Answer from the drawing. Dimensions are ordinates in mm from the lowest x, y and z of the part. Round coordinates to 2 decimals unless told otherwise and drop trailing zeros. Write each loop counter-clockwise with the first axis right and the second up, starting at its lowest first coordinate (ties: lowest second). Pieces come first, ordered by that corner, then holes. Notation, with made-up numbers: (1.5, 30) - (18.5, 30) arc R25 ccw to (18.5, 52) - close; hole circle Ø5 at (56.5, 75.5). An arc over 180 degrees is marked (long way). Answer in a Markdown table with one row per item.
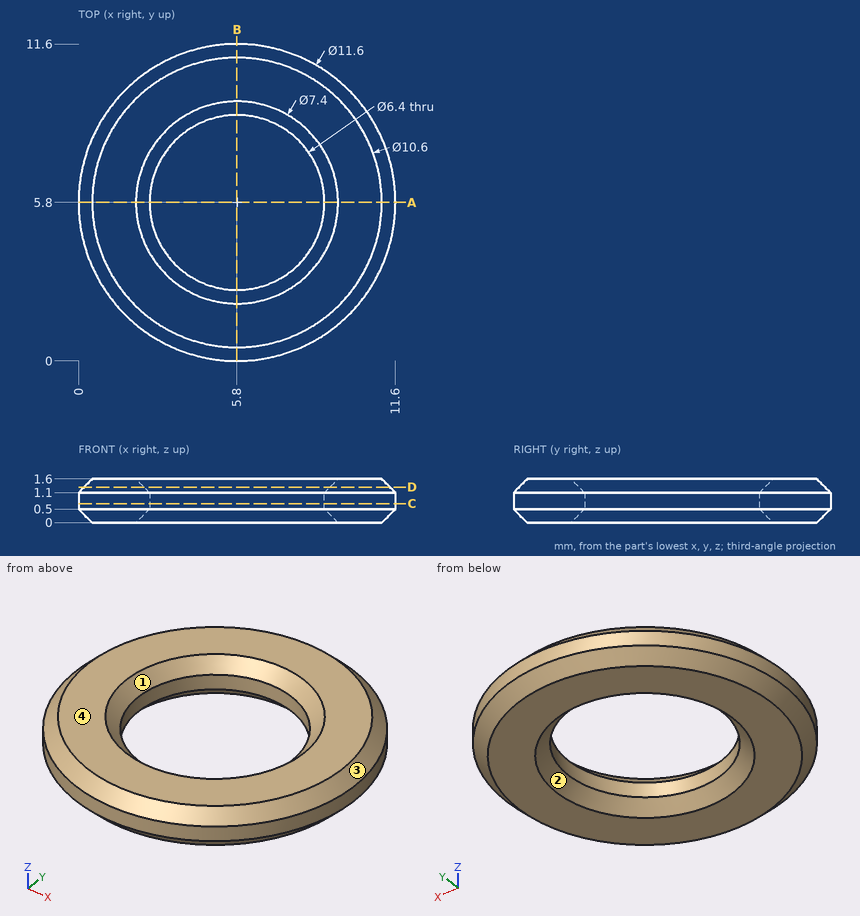
(1) For a pull along X with two mould halves and no side action, classify the marked faces 1, 2, 3 and 4 as pulls with the +X half, pulls with the -X half, needs draft (parallel to the pull), parting line crosses it, or undercut.
Checked values:
| item | result |
|---|---|
| face 1 | undercut |
| face 2 | undercut |
| face 3 | parting line crosses it |
| face 4 | needs draft |
(2) Section C-C (z = 0.7) is taken. Give the vertices of the cut face in (x, y).
Checked values:
| item | result |
|---|---|
| outline | circle Ø11.6 at (5.8, 5.8); hole circle Ø6.4 at (5.8, 5.8) |
(3) Section D-D (z = 1.3) is taken. Give the vertices of the cut face in (x, y), and give its area (3 significant figures).
Checked values:
| item | result |
|---|---|
| outline | circle Ø11.2 at (5.8, 5.8); hole circle Ø6.8 at (5.8, 5.8) |
| area | 62.2 mm2 |
(4) Section A-A (y = 5.8) is taken. Give the vertices of the cut face in (x, z).
Checked values:
| item | result |
|---|---|
| outline | (0, 0.5) - (0.5, 0) - (2.1, 0) - (2.6, 0.5) - (2.6, 1.1) - (2.1, 1.6) - (0.5, 1.6) - (0, 1.1) - close; (9, 0.5) - (9.5, 0) - (11.1, 0) - (11.6, 0.5) - (11.6, 1.1) - (11.1, 1.6) - (9.5, 1.6) - (9, 1.1) - close |
(5) Find the intervals of material crossed by line 1 (Y direction, x = 5.8, z = 0.7); line 2 (X direction, y = 6, z = 0.65); line 3 (Y direction, x = 3.5, z = 1.5), in increasing order.
Checked values:
| item | result |
|---|---|
| line 1 | y = 0 to 2.6, 9 to 11.6 |
| line 2 | x = 0 to 2.61, 8.99 to 11.6 |
| line 3 | y = 0.91 to 3.03, 8.57 to 10.69 |
